Read the model definition and answer for the solid it produces. Units are mm, in the model's axes. A direction names the side the tool comes from. Coordinates: 2 decimals unless noted, no trailing zeros. Write each loop counter-clockwise with the first axis right and the second up, starting at its lowest first coordinate (ties: lowest second). Pieces come first, ordered by that corner, then holes. Notation, with made-up numbers: M -17,18 L 26,18 A27 ccw 26,50 Z; hole C 5.25,-9.5 d10. An arc over 180 degrees is marked long. Write item = value, one per line.
from build123d import *

# Parameters (mm, degrees)
CROQUIS1_R              = 12.7
SALIENTE_EXTRUIR1_DEPTH = 3
CROQUIS2_R              = 4
SALIENTE_EXTRUIR2_DEPTH = 40
CROQUIS4_R              = 2
CORTAR_EXTRUIR1_DEPTH   = 10


with BuildPart() as part:
    # Croquis1 → Saliente-Extruir1 (new body)
    with BuildSketch(Plane(origin=(0, 0, 0), x_dir=(1, 0, 0), z_dir=(0, 1, 0))):
        with Locations(Location((0, 0, 0), (0, 0, 270))):
            Circle(CROQUIS1_R)
    extrude(amount=SALIENTE_EXTRUIR1_DEPTH)

    # Croquis2 → Saliente-Extruir2 (add)
    with BuildSketch(Plane.XZ):
        with Locations(Location((0, 0, 0), (0, 0, 270))):
            Circle(CROQUIS2_R)
    extrude(amount=SALIENTE_EXTRUIR2_DEPTH)

    # Croquis4 → Cortar-Extruir1 (cut)
    with BuildSketch(Plane(origin=(4, 0, 0), x_dir=(0, 0, -1), z_dir=(1, 0, 0))):
        with Locations((0, -36)):
            Circle(CROQUIS4_R)
    extrude(amount=-CORTAR_EXTRUIR1_DEPTH, mode=Mode.SUBTRACT)


solid = part.part
Item 1: Which of the six approach directions +Z, -Z, +X, -X, +Y, -Y give full straight-line access (tool end or side, diameter ignored) to faces 4 (the face through (-7.7, 1.5, -10.1)), 5 (the face through (-1.532, -19.72, -3.695))?
Worked answers:
face_4 = +Y, -Y
face_5 = -Y
Item 2: Find section C-C (y = -27). Determine the outline of the cut face in (x, z).
Worked answers:
outline = C 0,0 d8
Item 3: Consider line 1 along Y through (x, z) = (-0.25, 0); line 2 along Y through (x, z) = (0, 10.75); line 3 along X through (y, z) = (-21, 0). Determine where each line is inside the solid, lowest interval first. Write a range as from..to.
Worked answers:
line_1 = -40..-38, -34..3
line_2 = 0..3
line_3 = -4..4
Item 4: For a pull along Y with two mould halves and no side action, classify faces 1 (the face through (0, 3, 0)), 2 (the face through (3, 0, -3)), 3 (the face through (0.054, -36.766, -1.847)) as released by +Y, released by -Y, zero draft, split by the parting line, or undercut.
Worked answers:
face_1 = released by +Y
face_2 = released by -Y
face_3 = undercut
Item 5: Flat-ended cylindrical pins translate along their axes: pin 1 (10 mm diameter, centred on x = 8, y = -11.5, fed in from -Z); pin 2 (10 mm diameter, centred on x = 9, z = 3.5, fed in from -Y); pin 3 (1.5 mm diameter, centred on x = -1, y = -5, fed in from -Z); pin 4 (2.5 mm diameter, centred on y = -36, z = 0, fed in from -X). Find the tip coordinate at first contact, or state that the pin passes through.
Worked answers:
pin_1 = -2.65
pin_2 = 0
pin_3 = -3.99
pin_4 = through
Item 6: Find section A-A (z = 0). Determine the outline of the cut face in (x, y), and give its area (3 significant figures).
Worked answers:
outline = M -12.7,0 L -4,0 L -4,-34 L 4,-34 L 4,0 L 12.7,0 L 12.7,3 L -12.7,3 Z; M -4,-40 L 4,-40 L 4,-38 L -4,-38 Z
area = 364 mm²
Item 7: Find section D-D (y = -37). Determine the outline of the cut face in (x, z).
Worked answers:
outline = M -3.61,-1.73 A4 ccw 3.61,-1.73 Z; M -3.61,1.73 L 3.61,1.73 A4 ccw Z
Item 8: Find section B-B (x = 0). Determine the outline of the cut face in (y, z).
Worked answers:
outline = M -40,-4 L 0,-4 L 0,-12.7 L 3,-12.7 L 3,12.7 L 0,12.7 L 0,4 L -40,4 Z; hole C -36,0 d4
